from build123d import *

# Parameters (mm, degrees)
F1_DEPTH      = 2080
F2_W          = 32.756647
F2_H          = 43.48932
F2_H_2        = 26.490313
F3_DEPTH      = 25
F4_W          = 44.810192
F4_H          = 34.606159
F4_H_2        = 187.662824
F5_DEPTH      = 88.72009
F5_DEPTH_BACK = 90.01171
F6_W          = 27.187791
F6_H          = 22.711933
F6_H_2        = 20.19423
F7_DEPTH      = 25
F8_DEPTH      = 29.81951


with BuildPart() as f1:
    # F0 (on Right) → F1 (new body)
    with BuildSketch(Plane.YZ):
        with BuildLine():
            Line((22.995866, 145.190186), (0.938607, 5.92613))
            ThreePointArc((0.938607, 5.92613), (2.010635, 1.460812), (5.92613, -0.938607))
            Line((5.92613, -0.938607), (11.85226, -1.877214))
            ThreePointArc((11.85226, -1.877214), (16.317578, -0.805186), (18.716997, 3.11031))
            Line((18.716997, 3.11031), (40.774256, 142.374366))
            ThreePointArc((40.774256, 142.374366), (43.141482, 152.835998), (46.853973, 162.899144))
            Line((46.853973, 162.899144), (150.16508, 394.939691))
            ThreePointArc((150.16508, 394.939691), (182.336947, 493.954517), (193.219442, 597.494539))
            Line((193.219442, 597.494539), (193.219442, 616.494539))
            ThreePointArc((193.219442, 616.494539), (191.462083, 620.737179), (187.219442, 622.494539))
            Line((187.219442, 622.494539), (181.219442, 622.494539))
            ThreePointArc((181.219442, 622.494539), (176.976802, 620.737179), (175.219442, 616.494539))
            Line((175.219442, 616.494539), (175.219442, 597.494539))
            ThreePointArc((175.219442, 597.494539), (164.730291, 497.696927), (133.721262, 402.26095))
            Line((133.721262, 402.26095), (30.410155, 170.220404))
            ThreePointArc((30.410155, 170.220404), (25.882727, 157.948274), (22.995866, 145.190186))
        make_face()
    extrude(amount=F1_DEPTH)

    # F2 (on face) → F3 (cut)
    with BuildSketch(Plane(origin=(0, 0, 0), x_dir=(1, 0, 0), z_dir=(0, -0.987688, 0.156434))):
        with Locations((1.621677, -3.971665)):
            Rectangle(F2_W, F2_H)
        with Locations((1.621677, 151.018151)):
            Rectangle(F2_W, F2_H_2)
        with Locations((2078.378324, 151.018151)):
            Rectangle(F2_W, F2_H_2)
        with Locations((2078.378324, -3.971665)):
            Rectangle(F2_W, F2_H)
    extrude(amount=-F3_DEPTH, mode=Mode.SUBTRACT)

    # F4 (on face) → F5 (cut, two sides)
    with BuildSketch(Plane(origin=(0, -37.869946, 16.860786), x_dir=(1, 0, 0), z_dir=(0, -0.913545, 0.406737))) as f5_sk:
        with Locations((-4.405096, 166.424588)):
            Rectangle(F4_W, F4_H)
        with Locations((-4.405096, 497.559079)):
            Rectangle(F4_W, F4_H_2)
        with Locations((2084.405096, 497.559079)):
            Rectangle(F4_W, F4_H_2)
        with Locations((2084.405096, 166.424588)):
            Rectangle(F4_W, F4_H)
    extrude(amount=F5_DEPTH, mode=Mode.SUBTRACT)
    extrude(f5_sk.sketch, amount=-F5_DEPTH_BACK, mode=Mode.SUBTRACT)

    # F6 (on face) → F7 (cut)
    with BuildSketch(Plane.XZ.offset(-175.219442)):
        with Locations((4.406105, 562.20141)):
            Rectangle(F6_W, F6_H)
        with Locations((4.406105, 626.591654)):
            Rectangle(F6_W, F6_H_2)
        with Locations((2075.593896, 562.20141)):
            Rectangle(F6_W, F6_H)
        with Locations((2075.593896, 626.591654)):
            Rectangle(F6_W, F6_H_2)
    extrude(amount=-F7_DEPTH, mode=Mode.SUBTRACT)

    # F6 (on face) → F8 (cut)
    with BuildSketch(Plane.XZ.offset(-175.219442)):
        with Locations((4.406105, 562.20141)):
            Rectangle(F6_W, F6_H)
        with Locations((4.406105, 626.591654)):
            Rectangle(F6_W, F6_H_2)
        with Locations((2075.593896, 562.20141)):
            Rectangle(F6_W, F6_H)
        with Locations((2075.593896, 626.591654)):
            Rectangle(F6_W, F6_H_2)
    extrude(amount=F8_DEPTH, mode=Mode.SUBTRACT)


solid = f1.part
Here's how the part is built. I have some questions about the finished solid (model axes, mm). Coordinates: 2 decimals unless noted, no trailing zeros. Order: outer loops, then holes, each group sorted by start corner. A loop starts at its lowest first (then second) coordinate and runs counter-clockwise, first axis right, second up. Notation, with made-up numbers: (-16, 36) -> (40, 36) arc R20 ccw to (40, 44) -> close; hole circle Ø2 at (32.25, -12.5). An arc over 180 degrees is marked (long way). Answer in a Markdown table with one row per item.
(1) I want a section at A-A on x = 692.5. List the corners of the cut face in (y, z) for me, then the cut area to 3 significant figures.
Answer key:
| item | result |
|---|---|
| outline | (0.94, 5.93) arc R6 ccw to (5.93, -0.94) -> (11.85, -1.88) arc R6 ccw to (18.72, 3.11) -> (40.77, 142.37) arc R82 cw to (46.85, 162.9) -> (150.17, 394.94) arc R498 ccw to (193.22, 597.49) -> (193.22, 616.49) arc R6 ccw to (187.22, 622.49) -> (181.22, 622.49) arc R6 ccw to (175.22, 616.49) -> (175.22, 597.49) arc R480 cw to (133.72, 402.26) -> (30.41, 170.22) arc R100 ccw to (23, 145.19) -> close |
| area | 11,800 mm^2 |
(2) I want a section at C-C on z = 111. List the corners of the cut face in (x, y) for me.
Answer key:
| item | result |
|---|---|
| outline | (0, 17.58) -> (2080, 17.58) -> (2080, 35.81) -> (0, 35.81) -> close |
(3) Please list where these lines run through material, in increasing order: probe 1 along Y at (x, z) = (1053.5, 547); probe 2 along Y at (x, z) = (997, 162); probe 3 along X at (y, z) = (168, 506).
Answer key:
| item | result |
|---|---|
| probe 1 | 172.56 to 190.65 |
| probe 2 | 27.18 to 46.46 |
| probe 3 | 18 to 2062 |
(4) Thinking about a two-plate mould opening in X: for faces 1 (the face through (1025.44, 165.02, 499.07)), 2 (the face through (2080, 90, 282)), 3 (the face through (0, 21, 76)), which applies, +X half, -X half, draft (parallel to the pull), parting line (faces both ways), or undercut?
Answer key:
| item | result |
|---|---|
| face 1 | draft |
| face 2 | +X half |
| face 3 | -X half |
(5) I want a section at B-B on y = 106. List the corners of the cut face in (x, z) for me.
Answer key:
| item | result |
|---|---|
| outline | (0, 295.74) -> (2080, 295.74) -> (2080, 340) -> (0, 340) -> close |
(6) Will these pins go through, and if not, where does the flat tip stop? pin 1 Ø7 at (y, z) = (37, 152) entering from -X; pin 2 Ø2 at (x, z) = (1248, 523.5) entering from +Y; pin 3 Ø1.8 at (y, z) = (186, 620.5) entering from +X.
Answer key:
| item | result |
|---|---|
| pin 1 | x = 18 |
| pin 2 | y = 187.84 |
| pin 3 | x = 2062 |
